Answer from the drawing. Dimensions are ordinates in mm from the lowest x, y and z of the part. A direction names the side the tool comes from. Round coordinates to 2 decimals unless told otherwise and drop trailing zeros. Write each loop counter-clockwise with the first axis right and the second up, starting at its lowest first coordinate (ties: lowest second). Pieces come first, ordered by that corner, then holes. Notation, with made-up numbers: (76.5, 6.5) -> (102.5, 6.5) arc R14 ccw to (102.5, 22.5) -> close; hole circle Ø2 at (3, -36). An arc over 180 degrees is marked (long way). Return JSON: item names as keys, results as strings. Group by question number.
(1) A cutting plane is placed at B-B on y = 16.5. Give the vertices of the cut face in (x, z).
(2) For the marked faces 1, 2, 3 and 4, determine the directions among +Z, -Z, +X, -X, +Y, -Y from which every point of the face is accessible in a straight line to the end or side of a thin tool.
(3) A cutting plane is placed at D-D on z = 11. Give the vertices of the cut face in (x, y) (3 decimals).
(4) Given pin 1 (3 mm diameter, centred on x = 19, y = 29, fed in from -Z); pin 2 (11 mm diameter, centred on x = 6, z = 16.5, fed in from +Y); pin 3 (2 mm diameter, centred on x = 7.5, y = 2.5, fed in from -Z), each flat-ended and moving along its own axis, determine where each tip first touches the part or whether it passes through.
(5) Straight lines are drawn through the part: line 1 (Z direction, x = 6, y = 2.05); line 2 (X direction, y = 11.5, z = 44); line 3 (Y direction, x = 13.25, z = 12.5). For each, find the intervals that lie inside material, in ascending order.
(6) A cutting plane is placed at A-A on z = 27. Give the vertices of the cut face in (x, y).
(7) A cutting plane is placed at C-C on x = 1.5. Give the vertices of the cut face in (y, z), then the cut area to 3 significant figures.
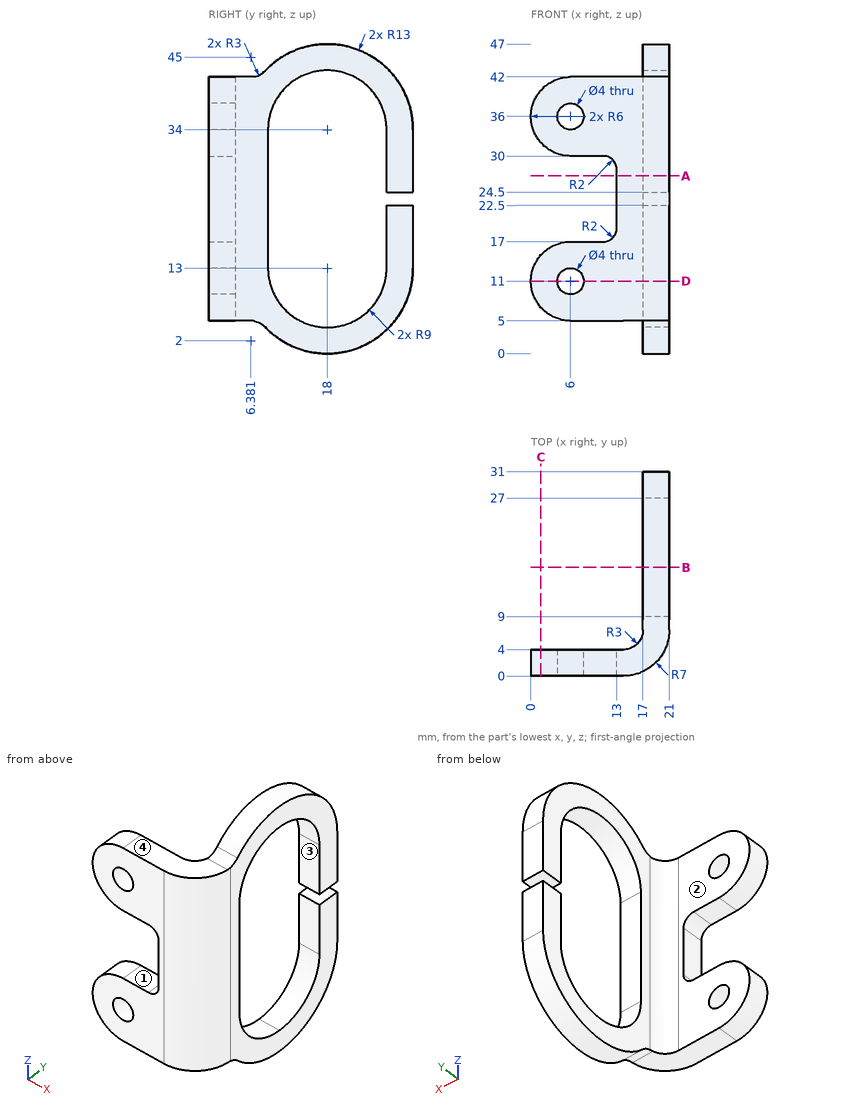
Checks:
{
 "1": {"outline": "(17, 0.09) -> (21, 0.09) -> (21, 4.13) -> (17, 4.13) -> close; (17, 42.87) -> (21, 42.87) -> (21, 46.91) -> (17, 46.91) -> close"},
 "2": {"face 1": "-X, +Y, -Y", "face 2": "+Z, -Z, -X, +Y", "face 3": "+X, -X", "face 4": "+Z, +X, -X, -Y"},
 "3": {"outline": "(0, 0) -> (4, 0) -> (4, 4) -> (0, 4) -> close; (8, 0) -> (14, 0) arc R7 ccw to (21, 7) -> (21, 9.225) -> (17, 9.225) -> (17, 7) arc R3 cw to (14, 4) -> (8, 4) -> close; (17, 26.775) -> (21, 26.775) -> (21, 30.845) -> (17, 30.845) -> close"},
 "4": {"pin 1": "stops at z = 4.13", "pin 2": "stops at y = 4", "pin 3": "stops at z = 5"},
 "5": {"line 1": "z = 5 to 9, 13 to 17, 30 to 34, 38 to 42", "line 2": "x = 17 to 21", "line 3": "y = 0 to 4"},
 "6": {"outline": "(13, 0) -> (14, 0) arc R7 ccw to (21, 7) -> (21, 9) -> (17, 9) -> (17, 7) arc R3 cw to (14, 4) -> (13, 4) -> close; (17, 27) -> (21, 27) -> (21, 31) -> (17, 31) -> close"},
 "7": {"outline": "(0, 7.03) -> (4, 7.03) -> (4, 14.97) -> (0, 14.97) -> close; (0, 32.03) -> (4, 32.03) -> (4, 39.97) -> (0, 39.97) -> close", "area": "63.5 mm^2"}
}
